```python
from build123d import *

# Parameters (mm, degrees)
BOSS_EXTRUDE1_DEPTH                                  = 60
FILLET1_R                                            = 3
SKETCH2_R                                            = 4.5
CUT_EXTRUDE1_DEPTH                                   = 8
TAP_DRILL_FOR_M3_TAP1_D                              = 2.7
TAP_DRILL_FOR_M3_TAP2_D                              = 2.5
CSK_FOR_M5_COUNTERSUNK_RAISED_HEAD_SCREW_D           = 5.3
CSK_FOR_M5_COUNTERSUNK_RAISED_HEAD_SCREW_CSINK_D     = 10.4
CSK_FOR_M5_COUNTERSUNK_RAISED_HEAD_SCREW_CSINK_ANGLE = 90


with BuildPart() as part:
    # Sketch1 → Boss-Extrude1 (new body)
    with BuildSketch(Plane.XY):
        Polygon((-4, 7), (-26, 7), (-26, 0), (26, 0), (26, 7), (4, 7), (4, 54), (-4, 54), align=None)
    extrude(amount=BOSS_EXTRUDE1_DEPTH)

    # Fillet1
    fillet1_edges = [part.edges().sort_by_distance(p)[0] for p in [
        (0, 54, 0),
        (26, 3.5, 0),
        (-26, 3.5, 0),
        (26, 3.5, 60),
        (-4, 7, 30),
        (4, 7, 30),
        (0, 54, 60),
        (-26, 3.5, 60),
    ]]
    fillet(fillet1_edges, radius=FILLET1_R)

    # Sketch2 → Cut-Extrude1 (cut)
    with BuildSketch(Plane(origin=(4, 0, 0), x_dir=(0, 0, -1), z_dir=(1, 0, 0))):
        with Locations(Location((-30, 25.5, 0), (0, 0, 90))):
            Circle(SKETCH2_R)
    extrude(amount=-CUT_EXTRUDE1_DEPTH, mode=Mode.SUBTRACT)

    # Tap Drill for M3 Tap1 (through all)
    with Locations(Plane(origin=(4, 25.5, 46.215), x_dir=(0, 1, 0), z_dir=(1, 0, 0))):
        with Locations((0, 0), (0, -32.43), (0, 6.7975), (0, -39.2275)):
            Hole(TAP_DRILL_FOR_M3_TAP1_D / 2)

    # Tap Drill for M3 Tap2 (through all)
    with Locations(Plane(origin=(4, 41.25, 40.48), x_dir=(0, 0, 1), z_dir=(1, 0, 0))):
        with Locations((0, 0), (-20.96, 0), (-19.460256121, 24.730256121), (-1.499743879, 24.730256121)):
            Hole(TAP_DRILL_FOR_M3_TAP2_D / 2)

    # CSK for M5 Countersunk Raised Head Screw1 (through all)
    with Locations(Plane(origin=(-15, 7, 16), x_dir=(1, 0, 0), z_dir=(0, 1, 0))):
        with Locations((0, 0), (0, -28), (30, -28), (30, 0)):
            CounterSinkHole(CSK_FOR_M5_COUNTERSUNK_RAISED_HEAD_SCREW_D / 2, CSK_FOR_M5_COUNTERSUNK_RAISED_HEAD_SCREW_CSINK_D / 2, counter_sink_angle=CSK_FOR_M5_COUNTERSUNK_RAISED_HEAD_SCREW_CSINK_ANGLE)


solid = part.part
```
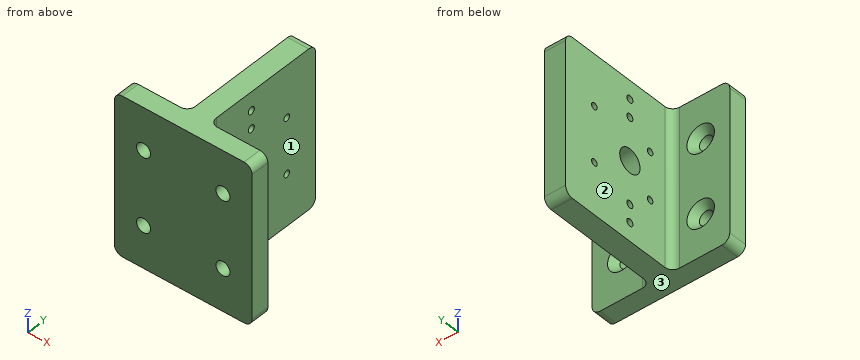
Input: part model. Units: mm. Frame: model coordinates. Face numbers are marked on the shaded views. A direction names the side the tool comes from. Coordinates: 2 decimals unless noted, no trailing zeros. Write each loop counter-clockwise with the first axis right and the second up, starting at its lowest first coordinate (ties: lowest second). Pieces come first, ordered by that corner, then holes.
1) Section A-A on y = 41.25. Output: boundary loops of the cut face in (x, z).
2) Section D-D on z = 44. Output: boundary loops of the cut face in (x, y).
3) Set-up query: the marked faces 1, 2 and 3. Return all of +Z, -Z, +X, -X, +Y, -Y with unobstructed straight access to the full face (end or side cutting, diameter ignored); none if empty.
4) Section B-B on z = 30. Output: boundary loops of the cut face in (x, y).
5) Material intervals for line 1 along X through (y, z) = (3, 44); line 2 along Z through (x, y) = (1.5, 16.5); line 3 along Z through (x, y) = (-15, 3.3), sorted ascending.
6) Pin query (flat end, axial travel): pin 1 Ø3 at (y, z) = (41.5, 10) entering from -X; pin 2 Ø8.5 at (x, z) = (15, 16) entering from +Y; pin 3 Ø5.5 at (x, z) = (16.5, 21.5) entering from +Y. Return the tip coordinate at first contact, or that it passes through.
7) Section C-C on x = 15. Output: boundary loops of the cut face in (y, z).
Check result:
1. outline: (-4, 0) - (4, 0) - (4, 18.27) - (-4, 18.27) - close; (-4, 20.77) - (4, 20.77) - (4, 39.23) - (-4, 39.23) - close; (-4, 41.73) - (4, 41.73) - (4, 60) - (-4, 60) - close
2. outline: (-26, 0) - (-17.65, 0) - (-17.65, 4.45) - (-20.2, 7) - (-26, 7) - close; (-12.35, 0) - (12.35, 0) - (12.35, 4.45) - (9.8, 7) - (7, 7) arc R3 cw to (4, 10) - (4, 54) - (-4, 54) - (-4, 10) arc R3 cw to (-7, 7) - (-9.8, 7) - (-12.35, 4.45) - close; (17.65, 0) - (26, 0) - (26, 7) - (20.2, 7) - (17.65, 4.45) - close
3. face 1: +Z, -Z, +X, +Y
3. face 2: +Z, -Z, -X, +Y
3. face 3: -Z, +X, -X, +Y, -Y
4. outline: (-26, 0) - (26, 0) - (26, 7) - (7, 7) arc R3 cw to (4, 10) - (4, 21) - (-4, 21) - (-4, 10) arc R3 cw to (-7, 7) - (-26, 7) - close; (-4, 30) - (4, 30) - (4, 54) - (-4, 54) - close
5. line 1: x = -26 to -17.65, -12.35 to 12.35, 17.65 to 26
5. line 2: z = 0 to 19.77, 22.27 to 37.73, 40.23 to 60
5. line 3: z = 0 to 13.35, 18.65 to 41.35, 46.65 to 60
6. pin 1: stops at x = -4
6. pin 2: stops at y = 6.05
6. pin 3: stops at y = 7
7. outline: (0, 0) - (7, 0) - (7, 10.8) - (4.45, 13.35) - (0, 13.35) - close; (0, 18.65) - (4.45, 18.65) - (7, 21.2) - (7, 38.8) - (4.45, 41.35) - (0, 41.35) - close; (0, 46.65) - (4.45, 46.65) - (7, 49.2) - (7, 60) - (0, 60) - close
